Design review of the part shown in the three views and the two pictorial views. Dimensions are in mm from the part's minimum x, y and z. A direction names the side the tool comes from. Round coordinates to 2 decimals unless told otherwise and drop trailing zeros. Order: outer loops, then holes, each group sorted by start corner. A loop starts at its lowest first (then second) coordinate and runs counter-clockwise, first axis right, second up. Notation, with made-up numbers: (22.25, -37) - (66.25, -37) arc R27 cw to (66.25, -2) - close; hole circle Ø8 at (7, -13.75). An arc over 180 degrees is marked (long way). One line per item, written item: value.
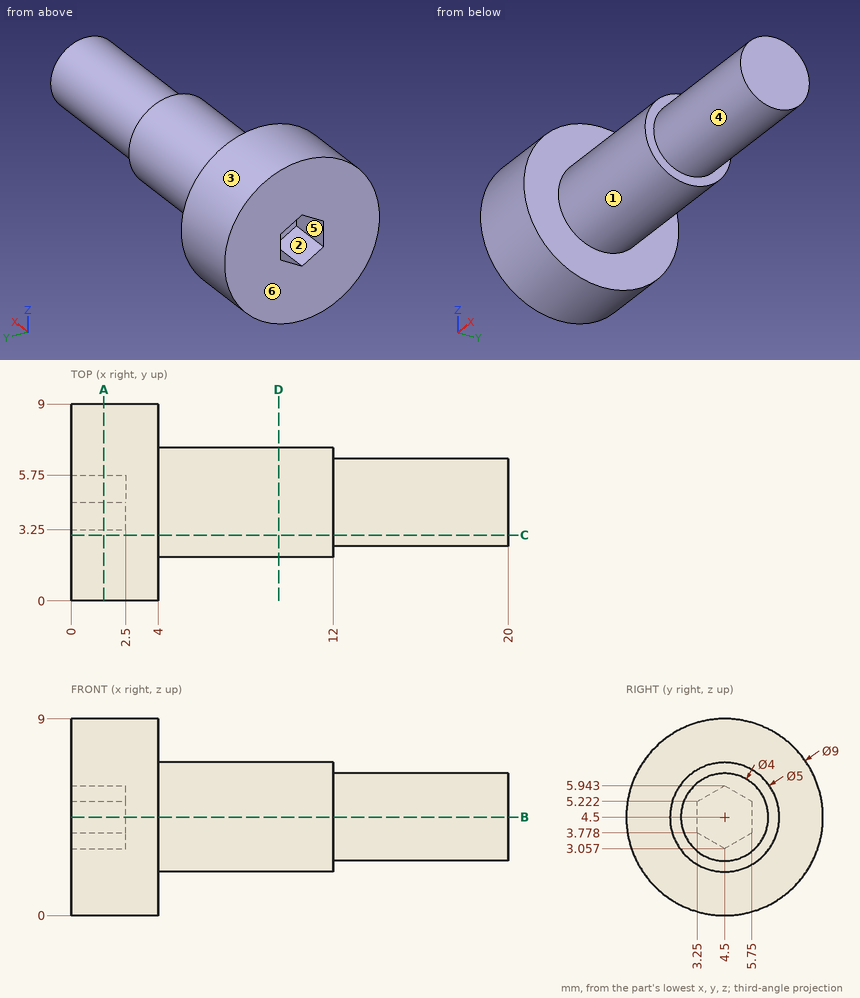
Item 1: Take a section at A-A (x = 1.5). Write out the cut boundary in (y, z).
Returned:
outline: circle Ø9 at (4.5, 4.5); hole (3.25, 3.78) - (4.5, 3.06) - (5.75, 3.78) - (5.75, 5.22) - (4.5, 5.94) - (3.25, 5.22) - close
Item 2: Machinability: for the marked faces 1, 2 and 3, which of the approach directions +Z, -Z, +X, -X, +Y, -Y give a long, thin tool a straight path to every point of the face, cutting with its end or side? Answer none if there is none.
Returned:
face 1: +X
face 2: -X
face 3: +X, -X
Item 3: The part is to be moulded in two halves that separate along Z. For the marked faces 4, 5 and 6, say which applies: +Z half, -Z half, draft (parallel to the pull), parting line (faces both ways), or undercut.
Returned:
face 4: parting line
face 5: undercut
face 6: draft
Item 4: Wall thickness on line 1 (X direction, y = 8.75, z = 3.5); line 2 (Y direction, x = 9.25, z = 4.5); line 3 (Z direction, x = 11, y = 6.25) (1 decimal): over which ranges is each line inside the solid? List them lowest first.
Returned:
line 1: 0 to 4
line 2: 2 to 7
line 3: 2.7 to 6.3
Item 5: For P1, Ø5, axis at x = 14.5, z = 8, coming from the +Y side; P2, Ø5, axis at x = 5.5, z = 7, coming from the +Y side; P3, Ø1, axis at y = 7, z = 7.5, coming from the +X side, all flat-tipped, find the tip position at first contact; note any pin that passes through.
Returned:
P1: y = 6.23
P2: y = 8.97
P3: x = 4
Item 6: Take a section at D-D (x = 9.5). Write out the cut boundary in (y, z), plus the area to 3 significant figures.
Returned:
outline: circle Ø5 at (4.5, 4.5)
area: 19.6 mm^2
Item 7: Take a section at C-C (y = 3). Write out the cut boundary in (x, z).
Returned:
outline: (0, 0.26) - (4, 0.26) - (4, 2.5) - (12, 2.5) - (12, 3.18) - (20, 3.18) - (20, 5.82) - (12, 5.82) - (12, 6.5) - (4, 6.5) - (4, 8.74) - (0, 8.74) - close
Item 8: Take a section at B-B (z = 4.5). Write out the cut boundary in (x, y).
Returned:
outline: (0, 0) - (4, 0) - (4, 2) - (12, 2) - (12, 2.5) - (20, 2.5) - (20, 6.5) - (12, 6.5) - (12, 7) - (4, 7) - (4, 9) - (0, 9) - (0, 5.75) - (2.5, 5.75) - (2.5, 3.25) - (0, 3.25) - close
